from build123d import *

# Parameters (mm, degrees)
EXTRUDE_1_DEPTH          = 5
SKETCH_2_R               = 25
CUT_EXTRUDE_1_DEPTH      = 5
SKETCH_3_R               = 1.5
CUT_EXTRUDE_2_DEPTH      = 5
PATTERN_CIRCULAR_1_COUNT = 3
SKETCH_5_R               = 1.5
CUT_EXTRUDE_3_DEPTH      = 13
PATTERN_CIRCULAR_2_COUNT = 8


with BuildPart() as part:
    # 草图1 → 凸台-拉伸1 (new body)
    with BuildSketch(Plane(origin=(0, 0, 0), x_dir=(1, 0, 0), z_dir=(0, 1, 0))):
        Polygon((36.084391824, 62.5), (-36.084391824, 62.5), (-72.168783649, 0), (-36.084391824, -62.5), (36.084391824, -62.5), (72.168783649, 0), align=None)
    extrude(amount=EXTRUDE_1_DEPTH)

    # 草图2 → 切除-拉伸1 (cut)
    with BuildSketch(Plane(origin=(0, 5, 0), x_dir=(1, 0, 0), z_dir=(0, 1, 0))):
        with Locations(Location((0, 0, 0), (0, 0, 270))):
            Circle(SKETCH_2_R)
    extrude(amount=-CUT_EXTRUDE_1_DEPTH, mode=Mode.SUBTRACT)

    # 草图3 → 切除-拉伸2 (cut)
    with BuildSketch(Plane(origin=(0, 5, 0), x_dir=(1, 0, 0), z_dir=(0, 1, 0))):
        with Locations(Location((-4.95, -45.05, 0), (0, 0, 270))):
            Circle(SKETCH_3_R)
        with Locations(Location((4.95, -45.05, 0), (0, 0, 270))):
            Circle(SKETCH_3_R)
        with Locations(Location((-4.95, -54.95, 0), (0, 0, 270))):
            Circle(SKETCH_3_R)
        with Locations(Location((4.95, -54.95, 0), (0, 0, 270))):
            Circle(SKETCH_3_R)
    cut_extrude_2 = extrude(amount=-CUT_EXTRUDE_2_DEPTH, mode=Mode.SUBTRACT)

    # 阵列(圆周)1: 切除-拉伸2 ×3 about axis
    pattern_circular_1_axis = Axis((0, 0, 0), (0, 1, 0))
    for i in range(1, PATTERN_CIRCULAR_1_COUNT):
        add(cut_extrude_2.rotate(pattern_circular_1_axis, i * 360 / PATTERN_CIRCULAR_1_COUNT), mode=Mode.SUBTRACT)

    # 草图5 → 切除-拉伸3 (cut)
    with BuildSketch(Plane.XZ):
        with Locations(Location((0, 30, 0), (0, 0, 270))):
            Circle(SKETCH_5_R)
    cut_extrude_3 = extrude(amount=-CUT_EXTRUDE_3_DEPTH, mode=Mode.SUBTRACT)

    # 阵列(圆周)2: 切除-拉伸3 ×8 about axis
    pattern_circular_2_axis = Axis((0, 0, 0), (0, 1, 0))
    for i in range(1, PATTERN_CIRCULAR_2_COUNT):
        add(cut_extrude_3.rotate(pattern_circular_2_axis, i * 360 / PATTERN_CIRCULAR_2_COUNT), mode=Mode.SUBTRACT)


solid = part.part
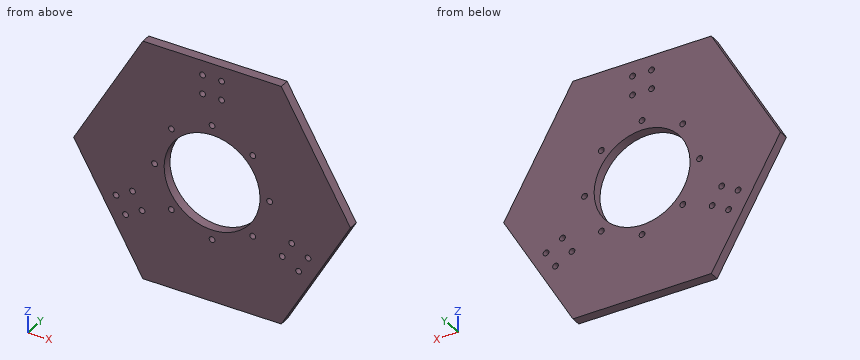
Source: CAD feature listing. Evaluate the final solid. Frame: model axes, mm. Give positions to 0.01 mm unless a question says otherwise; leave off trailing zeros. Loops run counter-clockwise (first coordinate to the right, second up) from the corner with the lowest first, then second, coordinate; pieces in that order, holes last. Notation, with made-up numbers: (5.5, 12.25) -> (14.5, 12.25) arc R25 cw to (14.5, 35.25) -> close; hole circle Ø9 at (10, 65). An arc over 180 degrees is marked (long way). Use a Markdown table: item, result. Add a question column.
1) First-contact query: pin 1 (5 mm diameter, centred on x = 45.11, z = -31.76, fed in from -Y); pin 2 (1.8 mm diameter, centred on x = 21.21, z = -21.21, fed in from +Y); pin 3 (2 mm diameter, centred on y = 1, z = -8, fed in from -X). Flat tips, straight axial feed; report the tip coordinate or a pass-through.
2) Line query: line 1 along X through (y, z) = (4.35, 55.5); line 2 along Z through (x, y) = (5, 2.4); line 3 along X through (y, z) = (1.9, -20.5). Output: solid intervals per line, ascending. Write a range as [from, to].
3) Section query A-A, the plane z = 6. Return the cut outline in (x, y), then the cut area to 3 significant figures.
4) Section query B-B, the plane y = 2.85. Count the separate pieces of the cut face and the enclosed holes in it, then the cut area to 3 significant figures.
Numbers:
| question | item | result |
|---|---|---|
| 1 | pin 1 | stops at y = 0 |
| 1 | pin 2 | passes through |
| 1 | pin 3 | stops at x = -68.13 |
| 2 | line 1 | x = [-40.13, -6.35], [-3.55, 3.55], [6.35, 40.13] |
| 2 | line 2 | z = [-62.5, -24.49], [24.49, 43.55], [46.55, 53.45], [56.45, 62.5] |
| 2 | line 3 | x = [-60.33, -22.53], [-19.89, -14.31], [14.31, 19.89], [22.53, 60.33] |
| 3 | outline | (-68.7, 0) -> (-24.27, 0) -> (-24.27, 5) -> (-68.7, 5) -> close; (24.27, 0) -> (68.7, 0) -> (68.7, 5) -> (24.27, 5) -> close |
| 3 | area | 444 mm2 |
| 4 | separate pieces | 1 |
| 4 | enclosed holes | 21 |
| 4 | area | 11,400 mm2 |
